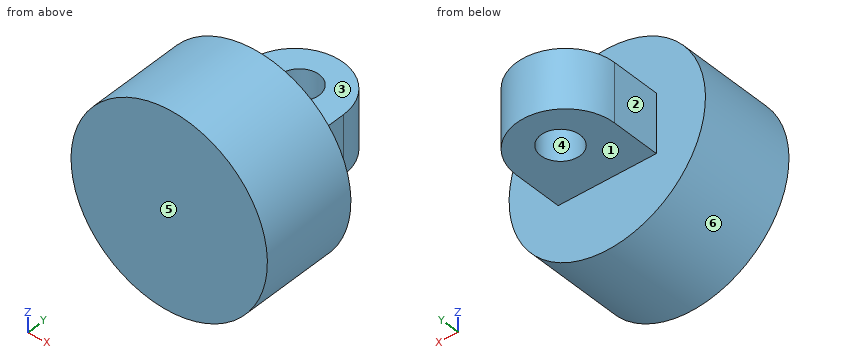
from build123d import *

# Parameters (mm, degrees)
CROQUIS1_R              = 50
SALIENTE_EXTRUIR1_DEPTH = 50
CROQUIS2_W              = 50
CROQUIS2_H              = 30
SALIENTE_EXTRUIR2_DEPTH = 50
CROQUIS3_R              = 10
CORTAR_EXTRUIR1_DEPTH   = 30
REDONDEO1_RADIUS        = 25
REDONDEO1_LENGTH        = 30


with BuildPart() as part:
    # Croquis1 → Saliente-Extruir1 (new body)
    with BuildSketch(Plane(origin=(0, 0, 0), x_dir=(1, 0, 0), z_dir=(0, 1, 0))):
        with Locations(Location((0, 0, 0), (0, 0, 270))):
            Circle(CROQUIS1_R)
    extrude(amount=SALIENTE_EXTRUIR1_DEPTH)

    # Croquis2 → Saliente-Extruir2 (add)
    with BuildSketch(Plane(origin=(0, 50, 0), x_dir=(1, 0, 0), z_dir=(0, 1, 0))):
        Rectangle(CROQUIS2_W, CROQUIS2_H)
    extrude(amount=SALIENTE_EXTRUIR2_DEPTH)

    # Croquis3 → Cortar-Extruir1 (cut)
    with BuildSketch(Plane(origin=(0, 0, -15), x_dir=(-1, 0, 0), z_dir=(0, 0, -1))):
        with Locations((0, 78)):
            Circle(CROQUIS3_R)
    extrude(amount=-CORTAR_EXTRUIR1_DEPTH, mode=Mode.SUBTRACT)

    # Redondeo1: full round fillet: the end face becomes a half cylinder, R = half its width
    redondeo1_face = Plane((0, 100, 0), x_dir=(0, 0, 1), z_dir=(0, 1, 0))  # on the end face: x along it, z out of the body
    redondeo1_slab = redondeo1_face.offset(-REDONDEO1_RADIUS / 2) * Box(REDONDEO1_LENGTH, 2 * REDONDEO1_RADIUS, REDONDEO1_RADIUS, mode=Mode.PRIVATE)  # the body's end, R deep
    redondeo1_round = Plane((0, 75, 0), x_dir=(0, 1, 0), z_dir=(0, 0, 1)) * Cylinder(REDONDEO1_RADIUS, REDONDEO1_LENGTH, mode=Mode.PRIVATE)  # its axis R under the face
    add(redondeo1_slab - redondeo1_round, mode=Mode.SUBTRACT)


solid = part.part
Verification items for the finished model (mm, model axes). Face numbers are marked on the shaded views. A direction names the side the tool comes from. Coordinates: 2 decimals unless noted, no trailing zeros. Order: outer loops, then holes, each group sorted by start corner. A loop starts at its lowest first (then second) coordinate and runs counter-clockwise, first axis right, second up.
1. Go/stop test with flat-tipped pins: pin 1 Ø23 at (x, y) = (0, 78) entering from +Z; pin 2 Ø4 at (y, z) = (15.5, -25) entering from -X; pin 3 Ø1 at (x, z) = (-20.5, -22.5) entering from +Y. Record where each tip stops, or that it passes through.
Results found:
pin 1: stops at z = 15
pin 2: stops at x = -44.4
pin 3: stops at y = 50
2. Sectioned sample at A-A, the plane z = 0. Record the cut outline in (x, y), and give its area (3 significant figures).
Results found:
outline: (-50, 0) - (50, 0) - (50, 50) - (25, 50) - (25, 75) arc R25 ccw to (-25, 75) - (-25, 50) - (-50, 50) - close; hole circle Ø20 at (0, 78)
area: 6,920 mm2
3. Scan lines: line 1 (Y direction, x = 0, z = -8); line 2 (Z direction, x = -17, y = 55.5); line 3 (Y direction, x = 33.5, z = -31). Record each from-to range of solid material in increasing order.
Results found:
line 1: y = 0 to 68, 88 to 100
line 2: z = -15 to 15
line 3: y = 0 to 50
4. Release check for a two-part mould opening along X. For the marked faces 4, 5 and 6 record: +X half, -X half, draft (parallel to the pull), parting line (faces both ways), or undercut.
Results found:
face 4: undercut
face 5: draft
face 6: parting line
5. Sectioned sample at D-D, the plane x = -13. Record the cut outline in (y, z), and give its area (3 significant figures).
Results found:
outline: (0, -48.28) - (50, -48.28) - (50, -15) - (96.35, -15) - (96.35, 15) - (50, 15) - (50, 48.28) - (0, 48.28) - close
area: 6,220 mm2
6. Set-up check for the marked faces 1, 2 and 3: record each of +Z, -Z, +X, -X, +Y, -Y from which the full face is reachable in a straight line by a thin tool's end or side.
Results found:
face 1: -Z, +X, -X, +Y
face 2: +Z, -Z, -X, +Y
face 3: +Z, +X, -X, +Y
7. Sectioned sample at C-C, the plane y = 84. Record the cut outline in (x, z).
Results found:
outline: (-23.32, -15) - (-8, -15) - (-8, 15) - (-23.32, 15) - close; (8, -15) - (23.32, -15) - (23.32, 15) - (8, 15) - close
8. Sectioned sample at B-B, the plane x = 0. Record the cut outline in (y, z).
Results found:
outline: (0, -50) - (50, -50) - (50, -15) - (68, -15) - (68, 15) - (50, 15) - (50, 50) - (0, 50) - close; (88, -15) - (100, -15) - (100, 15) - (88, 15) - close
